Source: CAD feature listing. Evaluate the final solid. Frame: model axes, mm. Round coordinates to 2 decimals unless told otherwise and drop trailing zeros. Loops run counter-clockwise (first coordinate to the right, second up) from the corner with the lowest first, then second, coordinate; pieces in that order, holes last. Notation, with made-up numbers: (76.25, 52) - (80.25, 52) arc R27 cw to (80.25, 91) - close; hole circle Ø2 at (24, 81). An arc over 180 degrees is marked (long way). One line per question, with ' | ' between items. Start each with the question number.
1. Cut plane B-B (x = -38.1). Return loops of the section in (y, z) (3 decimals).
2. Ray query, line 1 (Y direction, x = -38.1, z = 1.7) (3 decimals); line 2 (X direction, y = 38.1, z = 4.1) (3 decimals); line 3 (X direction, y = 44.5, z = 3.25). Return the intervals inside material, ascending.
3. Cut plane C-C (y = 39). Return loops of the section in (x, z), then the cut area to 3 significant figures.
4. Cut plane A-A (z = 1.1). Return loops of the section in (x, y) (3 decimals).
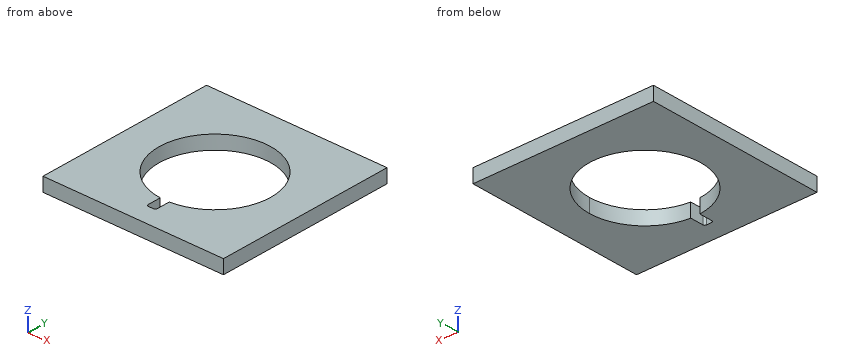
```python
from build123d import *

# Parameters (mm, degrees)
F0_W     = 76.2
F0_H     = 76.2
F1_DEPTH = 5.842
F3_DEPTH = 5.842


with BuildPart() as f1:
    # F0 (on Top) → F1 (new body)
    with BuildSketch(Plane.XY):
        with Locations((-38.1, 38.1)):
            Rectangle(F0_W, F0_H)
    extrude(amount=F1_DEPTH)

    # F2 (on face) → F3 (cut, through all)
    with BuildSketch(Plane.XY.offset(5.842)):
        with BuildLine():
            ThreePointArc((-36.195, 14.682357), (-38.1, 14.605), (-40.005, 14.682357))
            Line((-40.005, 14.682357), (-40.005, 9.017))
            ThreePointArc((-40.005, 9.017), (-39.781815, 8.478185), (-39.243, 8.255))
            Line((-39.243, 8.255), (-36.957, 8.255))
            ThreePointArc((-36.957, 8.255), (-36.418185, 8.478185), (-36.195, 9.017))
            Line((-36.195, 9.017), (-36.195, 14.682357))
        make_face()
        with BuildLine():
            Line((-40.005, 38.1), (-40.005, 14.682357))
            ThreePointArc((-40.005, 14.682357), (-38.1, 14.605), (-36.195, 14.682357))
            Line((-36.195, 14.682357), (-36.195, 38.1))
            Line((-36.195, 38.1), (-40.005, 38.1))
        make_face()
        with BuildLine():
            ThreePointArc((-36.195, 14.682357), (-20.826132, 22.174281), (-14.605, 38.1))
            ThreePointArc((-14.605, 38.1), (-54.025719, 55.373868), (-40.005, 14.682357))
            Line((-40.005, 14.682357), (-40.005, 38.1))
            Line((-40.005, 38.1), (-36.195, 38.1))
            Line((-36.195, 38.1), (-36.195, 14.682357))
        make_face()
    extrude(amount=-F3_DEPTH, mode=Mode.SUBTRACT)


solid = f1.part
```
Answers follow:
1) outline: (0, 0) - (8.255, 0) - (8.255, 5.842) - (0, 5.842) - close; (61.595, 0) - (76.2, 0) - (76.2, 5.842) - (61.595, 5.842) - close
2) line 1: y = 0 to 8.255, 61.595 to 76.2 | line 2: x = -76.2 to -61.595, -14.605 to 0 | line 3: x = -76.2 to -60.71, -15.49 to 0
3) outline: (-76.2, 0) - (-61.58, 0) - (-61.58, 5.84) - (-76.2, 5.84) - close; (-14.62, 0) - (0, 0) - (0, 5.84) - (-14.62, 5.84) - close | area: 171 mm2
4) outline: (-76.2, 0) - (0, 0) - (0, 76.2) - (-76.2, 76.2) - close; hole (-40.005, 9.017) arc R0.762 ccw to (-39.243, 8.255) - (-36.957, 8.255) arc R0.762 ccw to (-36.195, 9.017) - (-36.195, 14.682) arc R23.495 ccw (long way) to (-40.005, 14.682) - close
